```python
from build123d import *

# Parameters (mm, degrees)
SKETCH1_R                = 29.9847
SKETCH1_R_2              = 2.5527
BOSS_EXTRUDE1_DEPTH      = 2
BOSS_EXTRUDE2_DEPTH      = 2
FILLET1_R                = 1
CIRPATTERN1_COUNT        = 4
FILLET1_OF_CIRPATTERN1_R = 1


with BuildPart() as part:
    # Sketch1 → Boss-Extrude1 (new body)
    with BuildSketch(Plane.XY):
        Circle(SKETCH1_R)
        with Locations((-22.825356391, 7.416407865)):
            Circle(SKETCH1_R_2, mode=Mode.SUBTRACT)
        with Locations((-14.106846055, -19.416407865)):
            Circle(SKETCH1_R_2, mode=Mode.SUBTRACT)
        with Locations((14.106846055, -19.416407865)):
            Circle(SKETCH1_R_2, mode=Mode.SUBTRACT)
        with Locations((22.825356391, 7.416407865)):
            Circle(SKETCH1_R_2, mode=Mode.SUBTRACT)
        with Locations((0, 24)):
            Circle(SKETCH1_R_2, mode=Mode.SUBTRACT)
        with BuildLine():
            ThreePointArc((-10.931752655, 20.954613525), (-13.892128102, 19.120873957), (-16.550924391, 16.872046287))
            ThreePointArc((-16.550924391, 16.872046287), (-18.030688134, 13.903717203), (-17.363213066, 10.65484735))
            ThreePointArc((-17.363213066, 10.65484735), (-16.786147513, 5.454149951), (-20.309896586, 1.585887994))
            ThreePointArc((-20.309896586, 1.585887994), (-22.759533045, -0.650170928), (-23.307119088, -3.921382907))
            ThreePointArc((-23.307119088, -3.921382907), (-22.477935446, -7.303523957), (-21.160786474, -10.52711546))
            ThreePointArc((-21.160786474, -10.52711546), (-18.7950099, -12.851718542), (-15.498889917, -13.220868027))
            ThreePointArc((-15.498889917, -13.220868027), (-10.374409703, -14.279149951), (-7.78437231, -18.825793152))
            ThreePointArc((-7.78437231, -18.825793152), (-6.414733197, -21.846516076), (-3.472839121, -23.378161445))
            ThreePointArc((-3.472839121, -23.378161445), (0, -23.6347), (3.472839121, -23.378161445))
            ThreePointArc((3.472839121, -23.378161445), (6.414733197, -21.846516076), (7.78437231, -18.825793152))
            ThreePointArc((7.78437231, -18.825793152), (10.374409703, -14.279149951), (15.498889917, -13.220868027))
            ThreePointArc((15.498889917, -13.220868027), (18.7950099, -12.851718542), (21.160786474, -10.52711546))
            ThreePointArc((21.160786474, -10.52711546), (22.477935446, -7.303523957), (23.307119088, -3.921382907))
            ThreePointArc((23.307119088, -3.921382907), (22.759533045, -0.650170928), (20.309896586, 1.585887994))
            ThreePointArc((20.309896586, 1.585887994), (16.786147513, 5.454149951), (17.363213066, 10.65484735))
            ThreePointArc((17.363213066, 10.65484735), (18.030688134, 13.903717203), (16.550924391, 16.872046287))
            ThreePointArc((16.550924391, 16.872046287), (13.892128102, 19.120873957), (10.931752655, 20.954613525))
            ThreePointArc((10.931752655, 20.954613525), (7.651431793, 21.444688344), (4.767834088, 19.805925834))
            ThreePointArc((4.767834088, 19.805925834), (0, 17.65), (-4.767834088, 19.805925834))
            ThreePointArc((-4.767834088, 19.805925834), (-7.651431793, 21.444688344), (-10.931752655, 20.954613525))
        make_face(mode=Mode.SUBTRACT)
    extrude(amount=BOSS_EXTRUDE1_DEPTH)

    # Sketch1<4> → Boss-Extrude2 (add)
    with BuildSketch(Plane.XY):
        with BuildLine():
            Line((-3.355662517, 30.612532095), (-11.5, 33.770632582))
            Line((-11.5, 33.770632582), (-8.903800235, 28.632229663))
            ThreePointArc((-8.903800235, 28.632229663), (-4.502966651, 29.644654247), (0, 29.9847))
            ThreePointArc((0, 29.9847), (-1.706944937, 30.143008076), (-3.355662517, 30.612532095))
        make_face()
        with BuildLine():
            ThreePointArc((3.355662517, 30.612532095), (1.706944937, 30.143008076), (0, 29.9847))
            ThreePointArc((0, 29.9847), (4.502966651, 29.644654247), (8.903800235, 28.632229663))
            Line((8.903800235, 28.632229663), (11.5, 33.770632582))
            Line((11.5, 33.770632582), (3.355662517, 30.612532095))
        make_face()
    boss_extrude2 = extrude(amount=BOSS_EXTRUDE2_DEPTH)

    # Fillet1
    fillet1_edges = [part.edges().sort_by_distance(p)[0] for p in [
        (-8.903800235, 28.632229663, 1),
        (8.903800235, 28.632229663, 1),
    ]]
    fillet(fillet1_edges, radius=FILLET1_R)

    # CirPattern1: Boss-Extrude2 ×4 about axis
    cirpattern1_axis = Axis((0, 0, 0), (0, 0, 1))
    for i in range(1, CIRPATTERN1_COUNT):
        add(boss_extrude2.rotate(cirpattern1_axis, i * 360 / CIRPATTERN1_COUNT))

    # Fillet1 of CirPattern1
    fillet1_of_cirpattern1_edges = [part.edges().sort_by_distance(p)[0] for p in [
        (-28.632229663, -8.903800235, 1),
        (-28.632229663, 8.903800235, 1),
        (8.903800235, -28.632229663, 1),
        (-8.903800235, -28.632229663, 1),
        (28.632229663, 8.903800235, 1),
        (28.632229663, -8.903800235, 1),
    ]]
    fillet(fillet1_of_cirpattern1_edges, radius=FILLET1_OF_CIRPATTERN1_R)


solid = part.part
```
The listing builds one solid part. Answer for the finished solid, in the listing's coordinates (mm). A direction names the side the tool comes from. Coordinates: 2 decimals unless noted, no trailing zeros. Write each loop counter-clockwise with the first axis right and the second up, starting at its lowest first coordinate (ties: lowest second). Pieces come first, ordered by that corner, then holes. Notation, with made-up numbers: (37, -36.75) -> (73, -36.75) arc R11 cw to (73, -15.75) -> close; hole circle Ø9 at (-8.5, -16.75). An arc over 180 degrees is marked (long way). Write each question's results on one line, items separated by ' | '. Start each with the question number.
1) A flat-ended cylindrical pin translates along its axis: pin 1 Ø4 at (x, y) = (0, 24) entering from -Z. Find the tip coordinate at first contact, or state that the pin passes through.
2) A cutting plane is placed at C-C (x = -22). Determine the outline of the cut face in (y, z), then the cut area to 3 significant figures.
3) A cutting plane is placed at B-B (x = 12.5). Determine the outline of the cut face in (y, z).
4) A cutting plane is placed at D-D (z = 0.85). Count the separate pieces of the cut face and the enclosed holes in it, then the cut area to 3 significant figures.
5) A tool of negligible diameter and unlimited length cuts with its end or side. For faces 4 (the flat face through (-32.17, -7.37, 0.99)), 5 (the cylindrical face through (0.08, 17.65, 0.99)), 6 (the flat face through (31.69, -10.45, 0.99)), 7 (the flat face through (-31.69, 10.45, 0.99)), from which of +Z, -Z, +X, -X, +Y, -Y can it reach the whole face along a straight path? Write none if from no direction.
6) A cutting plane is placed at A-A (y = -18). Determine the outline of the cut face in (x, z), then the cut area to 3 significant figures.
7) Straight lines are drawn through the part: probe 1 along Y at (x, z) = (0, 0.8); probe 2 along Y at (x, z) = (-14, 1.2); probe 3 along X at (y, z) = (-10, 0.3). For each, find the intervals that lie inside material, in ascending order.
8) For a pull along X with two mould halves and no side action, classify faces 1 (the flat face through (-7.37, 32.17, 0.99)), 2 (the flat face through (0, 18, 2)), 3 (the flat face through (-10.45, -31.69, 0.99)) as +X half, -X half, draft (parallel to the pull), parting line (faces both ways), or undercut.
Values follow:
1) pin 1: through
2) outline: (-20.37, 0) -> (-8.64, 0) -> (-8.64, 2) -> (-20.37, 2) -> close; (0.4, 0) -> (5, 0) -> (5, 2) -> (0.4, 2) -> close; (9.83, 0) -> (20.37, 0) -> (20.37, 2) -> (9.83, 2) -> close | area: 53.8 mm²
3) outline: (-27.25, 0) -> (-21.4, 0) -> (-21.4, 2) -> (-27.25, 2) -> close; (-17.43, 0) -> (-13.27, 0) -> (-13.27, 2) -> (-17.43, 2) -> close; (20.06, 0) -> (27.25, 0) -> (27.25, 2) -> (20.06, 2) -> close
4) separate pieces: 1 | enclosed holes: 6 | area: 1,440 mm²
5) face 4: +Z, -Z, -X | face 5: +Z, -Z | face 6: +Z, -Z, -Y | face 7: +Z, -Z, +Y
6) outline: (-23.98, 0) -> (-16.23, 0) -> (-16.23, 2) -> (-23.98, 2) -> close; (-11.98, 0) -> (-7.92, 0) -> (-7.92, 2) -> (-11.98, 2) -> close; (7.92, 0) -> (11.98, 0) -> (11.98, 2) -> (7.92, 2) -> close; (16.23, 0) -> (23.98, 0) -> (23.98, 2) -> (16.23, 2) -> close | area: 47.3 mm²
7) probe 1: -29.98 to -23.63, 17.65 to 21.45, 26.55 to 29.98 | probe 2: -26.52 to -21.97, -16.87 to -13.07, 19.04 to 26.52 | probe 3: -33.19 to -30.8, -28.27 to -21.41, 21.41 to 28.27, 30.8 to 33.19
8) face 1: undercut | face 2: draft | face 3: -X half
